```python
from build123d import *
from build123d.topology import SkipClean

# Parameters (mm, degrees)
BOSS_EXTRUDE1_DEPTH      = 10
SKETCH4_R                = 1.962636903
CUT_EXTRUDE2_DEPTH       = 10
SKETCH6_R                = 2.5
SKETCH6_R_2              = 1.962636903
BOSS_EXTRUDE2_DEPTH      = 3.333333333
BOSS_EXTRUDE3_START      = -3.333333333
SKETCH7_R                = 2.5
SKETCH7_R_2              = 1.962636903
BOSS_EXTRUDE3_DEPTH      = 3.333333333
SKETCH9_W                = 3.333333334
SKETCH9_H                = 5
CUT_EXTRUDE7_DEPTH       = 3
SKETCH10_W               = 3.333333334
SKETCH10_H               = 1.037363097
CUT_EXTRUDE8_DEPTH       = 37.201372358
BOSS_EXTRUDE4_DEPTH      = 1.5
BOSS_EXTRUDE4_DEPTH_BACK = 1.5
SKETCH12_R               = 2
BOSS_EXTRUDE9_DEPTH      = 1.6
BOSS_EXTRUDE9_DEPTH_BACK = 1.6


with BuildPart() as part:
    # Sketch3 → Boss-Extrude1 (new body)
    with BuildSketch(Plane(origin=(0, 0, 0), x_dir=(0, 0, -1), z_dir=(1, 0, 0))):
        Polygon((30, 2.5), (31.962636903, 2.5), (31.97894003, 5), (30, 5), (0, 5), (0, 0), (30, 0), align=None)
    extrude(amount=BOSS_EXTRUDE1_DEPTH)

    # Sketch4 → Cut-Extrude2 (cut)
    with BuildSketch(Plane(origin=(0, 0, 0), x_dir=(0, 0, -1), z_dir=(1, 0, 0))):
        with Locations((31.962636903, 2.5)):
            Circle(SKETCH4_R)
    extrude(amount=CUT_EXTRUDE2_DEPTH, mode=Mode.SUBTRACT)

    # Sketch6 → Boss-Extrude2 (add)
    with BuildSketch(Plane.ZY):
        with Locations((-31.962636903, 2.5)):
            Circle(SKETCH6_R)
        with Locations((-31.962636903, 2.5)):
            Circle(SKETCH6_R_2, mode=Mode.SUBTRACT)
    extrude(amount=-BOSS_EXTRUDE2_DEPTH)

    # Sketch7 → Boss-Extrude3 (add)
    with BuildSketch(Plane(origin=(10, 0, 0), x_dir=(0, 0, -1), z_dir=(1, 0, 0)).offset(BOSS_EXTRUDE3_START)):
        with Locations((31.962636903, 2.5)):
            Circle(SKETCH7_R)
        with Locations((31.962636903, 2.5)):
            Circle(SKETCH7_R_2, mode=Mode.SUBTRACT)
    extrude(amount=BOSS_EXTRUDE3_DEPTH)

    # Sketch9 → Cut-Extrude7 (cut)
    with SkipClean():  # the faces are left unmerged after this step: merging them gives an invalid solid
        with BuildSketch(Plane(origin=(0, -0.208321197, -31.944975261), x_dir=(-1, 0, 0), z_dir=(0, -0.006521112201233067, -0.9999787373217788))):
            with Locations((-5, 2.708378785)):
                Rectangle(SKETCH9_W, SKETCH9_H)
        extrude(amount=-CUT_EXTRUDE7_DEPTH, mode=Mode.SUBTRACT)

    # Sketch10 → Cut-Extrude8 (cut, through all)
    with SkipClean():  # the faces are left unmerged after this step: merging them gives an invalid solid
        with BuildSketch(Plane(origin=(0, 0.208374354, -0.001358861), x_dir=(1, 0, 0), z_dir=(0, 0.9999787373217788, -0.00652111220123307))):
            with Locations((5, 29.464336059)):
                Rectangle(SKETCH10_W, SKETCH10_H)
        extrude(amount=-CUT_EXTRUDE8_DEPTH, mode=Mode.SUBTRACT)

    # Sketch12 → Boss-Extrude4 (add, two sides: drawn at the far end of the back side and taken through both)
    with SkipClean():  # the faces are left unmerged after this step: merging them gives an invalid solid
        with BuildSketch(Plane(origin=(5, 0, 0), x_dir=(0, 0, -1), z_dir=(1, 0, 0)).offset(-BOSS_EXTRUDE4_DEPTH_BACK)):
            with BuildLine():
                Line((-2.5, 5), (0, 5))
                Line((0, 5), (0, 2.5))
                ThreePointArc((0, 2.5), (-4.267766953, 0.732233047), (-2.5, 5))
            make_face()
            with Locations((-2.5, 2.5)):
                Circle(SKETCH12_R, mode=Mode.SUBTRACT)
        extrude(amount=BOSS_EXTRUDE4_DEPTH + BOSS_EXTRUDE4_DEPTH_BACK)

    # Sketch13 → Boss-Extrude9 (add, two sides: drawn at the far end of the back side and taken through both)
    with SkipClean():  # the faces are left unmerged after this step: merging them gives an invalid solid
        with BuildSketch(Plane(origin=(5, 0, 0), x_dir=(0, 0, -1), z_dir=(1, 0, 0)).offset(-BOSS_EXTRUDE9_DEPTH_BACK)):
            with BuildLine():
                Line((24.809137755, 5), (28, 5))
                Line((28, 5), (38, 5))
                Line((38, 5), (38, 6.25))
                Line((38, 6.25), (28, 6.25))
                add(Edge.make_bspline(
                    [(28, 6.25), (27.570139782, 6.25), (27.108034748, 5.787413316), (26.444737385, 5.323894947), (26.11400028, 5.04700236), (24.809137755, 5.04700236)],
                    knots=[0, 0, 0, 0, 0.435997525, 0.535997525, 1, 1, 1, 1], degree=3))
                Line((24.809137755, 5.04700236), (24.809137755, 5))
            make_face()
        extrude(amount=BOSS_EXTRUDE9_DEPTH + BOSS_EXTRUDE9_DEPTH_BACK)


solid = part.part
```
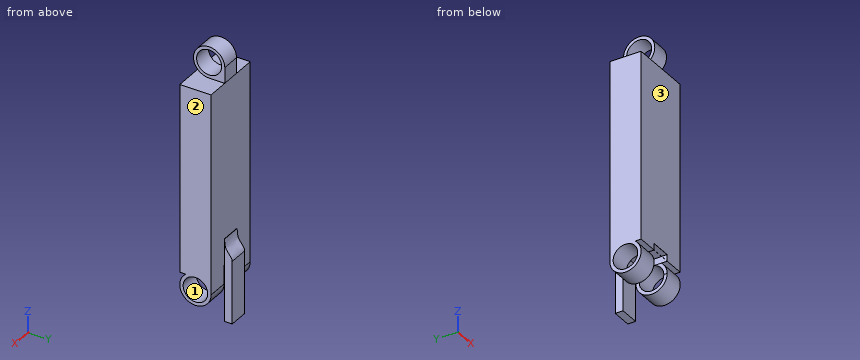
The listing builds one solid part. Answer for the finished solid, in the listing's coordinates (mm). Face numbers are marked on the shaded views. Round coordinates to 2 decimals unless told otherwise and drop trailing zeros. Loops run counter-clockwise (first coordinate to the right, second up) from the corner with the lowest first, then second, coordinate; pieces in that order, holes last. Notation, with made-up numbers: (37, -38) - (92, -38) arc R14 cw to (92, -19) - close; hole circle Ø10 at (-29, 70). An arc over 180 degrees is marked (long way). Use one line per item in the form item = value. Start each with the question number.
1. Consider line 1 (Y direction, x = 4.25, z = 2.5); line 2 (Z direction, x = 2, y = 2.5); line 3 (Y direction, x = 5, z = -14). Determine where each line is inside the solid, lowest interval first. Write a range as [from, to].
2. Given pin 1 Ø1 at (x, z) = (4.5, -34.5) entering from -Y; pin 2 Ø1 at (x, y) = (3, 0.5) entering from -Z; pin 3 Ø1.2 at (x, z) = (4.5, 1) entering from +Y; pin 4 Ø3.5 at (y, z) = (2.5, 2.5) entering from -X, each flat-ended and moving along its own axis, determine where each tip first touches the part or whether it passes through.
3. For a pull along Y with two mould halves and no side action, classify the marked faces 1, 2 and 3 as pulls with the +Y half, pulls with the -Y half, needs draft (parallel to the pull), parting line crosses it, or undercut.
4. The part is cut by section A-A on y = 1.75. Determine the outline of the cut face in (x, z).
5. The part is cut by section C-C on y = 4. Determine the outline of the cut face in (x, z).
6. The part is cut by section D-D on x = 4.25. Give the number of separate pieces and of enclosed holes in the cut face, then the cut area to 3 significant figures.
Geometry check:
q1.line_1 = [0, 0.5], [4.5, 5]
q1.line_2 = [-34.46, -33.93], [-30, 0]
q1.line_3 = [0, 5]
q2.pin_1 = 5
q2.pin_2 = -33.96
q2.pin_3 = 5
q2.pin_4 = through
q3.face_1 = undercut
q3.face_2 = needs draft
q3.face_3 = pulls with the -Y half
q4.outline = (0, -34.35) - (3.33, -34.35) - (3.33, -33.78) - (0, -33.78) - close; (0, -30.15) - (3.33, -30.15) - (3.33, -28.96) - (6.67, -28.96) - (6.67, -30.15) - (10, -30.15) - (10, 0) - (0, 0) - close; (3.5, 0.12) - (6.5, 0.12) - (6.5, 0.65) - (3.5, 0.65) - close; (3.5, 4.35) - (6.5, 4.35) - (6.5, 4.88) - (3.5, 4.88) - close; (6.67, -34.35) - (10, -34.35) - (10, -33.78) - (6.67, -33.78) - close
q5.outline = (0, -33.96) - (3.33, -33.96) - (3.33, -33.23) - (0, -33.23) - close; (0, -30.7) - (3.33, -30.7) - (3.33, -28.97) - (6.67, -28.97) - (6.67, -30.7) - (10, -30.7) - (10, 0) - (6.5, 0) - (6.5, 1.18) - (3.5, 1.18) - (3.5, 0) - (0, 0) - close; (3.5, 3.82) - (6.5, 3.82) - (6.5, 4.5) - (3.5, 4.5) - close; (6.67, -33.96) - (10, -33.96) - (10, -33.23) - (6.67, -33.23) - close
q6.separate_pieces = 2
q6.enclosed_holes = 1
q6.area = 167 mm^2
